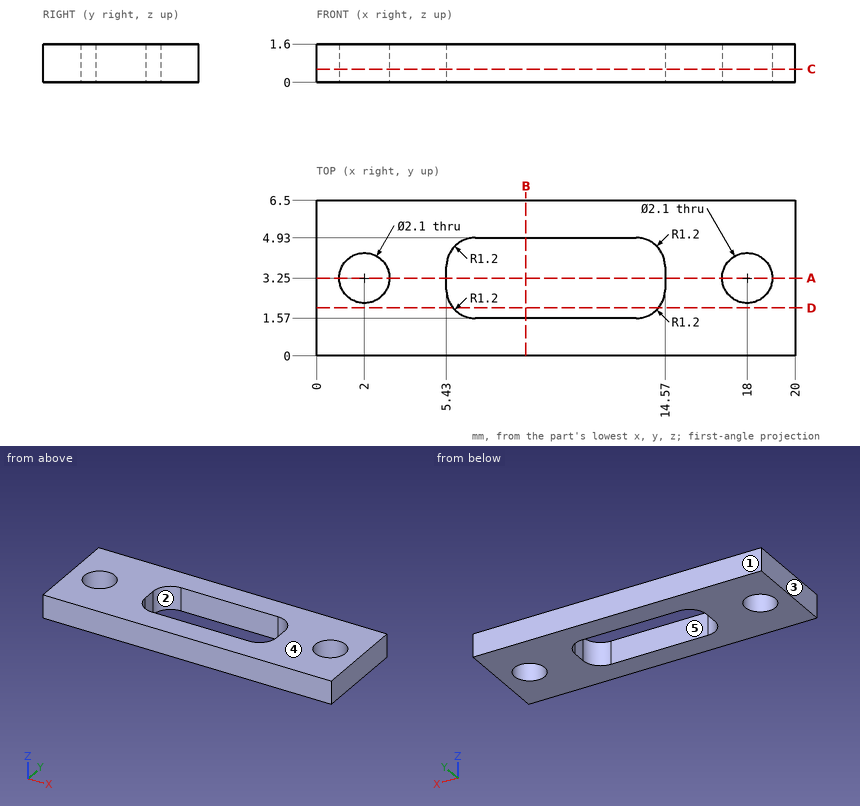
Input: dimensioned drawing with shaded views. Units: mm. Origin: part minimum x, y, z. A direction names the side the tool comes from. Coordinates: 2 decimals unless noted, no trailing zeros. Order: outer loops, then holes, each group sorted by start corner. A loop starts at its lowest first (then second) coordinate and runs counter-clockwise, first axis right, second up.
(1) Section query D-D (y = 2). Return the cut outline in (x, z).
(2) Section query C-C (z = 0.55). Return the cut outline in (x, y).
(3) Section query B-B (x = 8.75). Return the cut outline in (y, z).
(4) Access query for the marked faces 1 and 2. Directions: +Z, -Z, +X, -X, +Y, -Y. A direction counts if a zero-diameter tool reaches every point of the face in a straight line with its end or side. Return the directions, or none.
(5) Draft query along X for the marked faces 3, 4 and 5. Return one class per face: pulls with the +X half, pulls with the -X half, needs draft (parallel to the pull), parting line crosses it, or undercut.
(6) Section query A-A (y = 3.25). Return the cut outline in (x, z).
(7) Material intervals for probe 1 along X at (y, z) = (3.25, 0.9); probe 2 along Y at (x, z) = (2, 0.3); probe 3 along X at (y, z) = (2.5, 0.8), sorted ascending.
(8) First-contact query: pin 1 (3.5 mm diameter, centred on x = 2, y = 3.25, fed in from -Z); pin 2 (1.3 mm diameter, centred on x = 18, y = 3.25, fed in from -Z). Flat tips, straight axial feed; report the tip coordinate or a pass-through.
Solution:
1. outline: (0, 0) - (5.71, 0) - (5.71, 1.6) - (0, 1.6) - close; (14.29, 0) - (20, 0) - (20, 1.6) - (14.29, 1.6) - close
2. outline: (0, 0) - (20, 0) - (20, 6.5) - (0, 6.5) - close; hole circle Ø2.1 at (2, 3.25); hole (5.43, 2.77) arc R1.2 ccw to (6.63, 1.57) - (13.37, 1.57) arc R1.2 ccw to (14.57, 2.77) - (14.57, 3.73) arc R1.2 ccw to (13.37, 4.93) - (6.63, 4.93) arc R1.2 ccw to (5.43, 3.73) - close; hole circle Ø2.1 at (18, 3.25)
3. outline: (0, 0) - (1.57, 0) - (1.57, 1.6) - (0, 1.6) - close; (4.93, 0) - (6.5, 0) - (6.5, 1.6) - (4.93, 1.6) - close
4. face 1: +Z, -Z, +X, -X, +Y
4. face 2: +Z, -Z
5. face 3: pulls with the -X half
5. face 4: needs draft
5. face 5: undercut
6. outline: (0, 0) - (0.95, 0) - (0.95, 1.6) - (0, 1.6) - close; (3.05, 0) - (5.43, 0) - (5.43, 1.6) - (3.05, 1.6) - close; (14.57, 0) - (16.95, 0) - (16.95, 1.6) - (14.57, 1.6) - close; (19.05, 0) - (20, 0) - (20, 1.6) - (19.05, 1.6) - close
7. probe 1: x = 0 to 0.95, 3.05 to 5.43, 14.57 to 16.95, 19.05 to 20
7. probe 2: y = 0 to 2.2, 4.3 to 6.5
7. probe 3: x = 0 to 1.27, 2.73 to 5.46, 14.54 to 17.27, 18.73 to 20
8. pin 1: stops at z = 0
8. pin 2: passes through
